The drawing under review shows one solid part. Ordinate dimensions are in mm from its lowest x, y, z. Round coordinates to 2 decimals unless told otherwise and drop trailing zeros. Write each loop counter-clockwise with the first axis right and the second up, starting at its lowest first coordinate (ties: lowest second). Pieces come first, ordered by that corner, then holes. Notation, with made-up numbers: (-5, 62.5) -> (11, 62.5) arc R24 cw to (11, 92.5) -> close; hole circle Ø10 at (54.5, -3). An arc over 180 degrees is marked (long way). Answer in a Markdown table with one row per item.
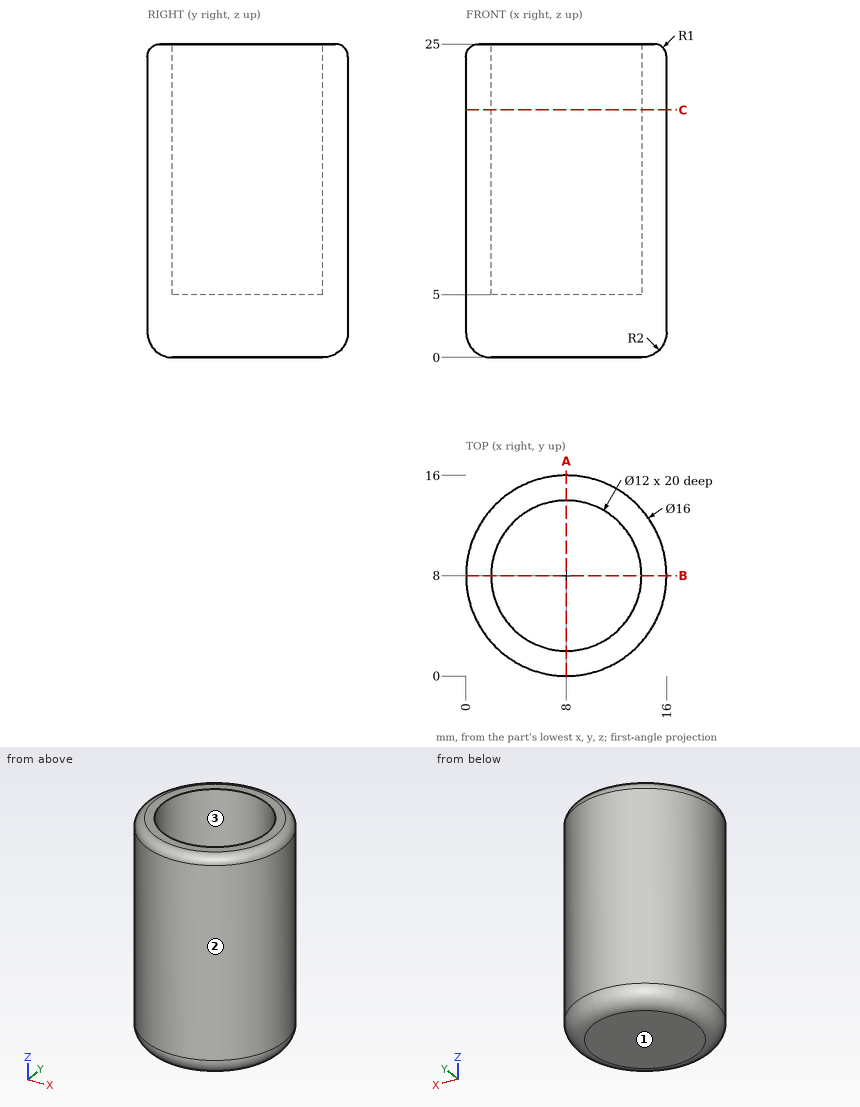
1) Mouldability with a two-part tool opening along Y and no side actions: class the marked faces 1, 2 and 3 as pulls with the +Y half, pulls with the -Y half, needs draft (parallel to the pull), parting line crosses it, or undercut.
Solved:
| item | result |
|---|---|
| face 1 | needs draft |
| face 2 | parting line crosses it |
| face 3 | undercut |
2) Clearance check with flat-ended pins moving along their axes: pin 1 Ø1.5 at (y, z) = (10.5, 10.5) entering from -X; pin 2 Ø5 at (x, y) = (2, 12) entering from -Z; pin 3 Ø6 at (x, z) = (13.5, 6) entering from +Y; pin 4 Ø2 at (x, z) = (14.5, 16.5) entering from +Y. State where each tip first meets the part, or that it passes through.
Solved:
| item | result |
|---|---|
| pin 1 | x = 0.19 |
| pin 2 | z = 0 |
| pin 3 | y = 15.6 |
| pin 4 | y = 13.81 |
3) Consider section A-A on x = 8. State the section outline as (y, z) points, then the cut area to 3 significant figures.
Solved:
| item | result |
|---|---|
| outline | (0, 2) arc R2 ccw to (2, 0) -> (14, 0) arc R2 ccw to (16, 2) -> (16, 24) arc R1 ccw to (15, 25) -> (14, 25) -> (14, 5) -> (2, 5) -> (2, 25) -> (1, 25) arc R1 ccw to (0, 24) -> close |
| area | 158 mm² |
4) For line 1 (Y direction, x = 8, z = 20.75); line 2 (Z direction, x = 4.5, y = 10); line 3 (Y direction, x = 13, z = 13.25) (3 decimals), list the stretches that pass through material, from the lowest coordinate up. Write a range as [from, to].
Solved:
| item | result |
|---|---|
| line 1 | [0, 2], [14, 16] |
| line 2 | [0, 5] |
| line 3 | [1.755, 4.683], [11.317, 14.245] |
5) Consider section C-C on z = 19.75. State the section outline as (x, y) points, then the cut area to 3 significant figures.
Solved:
| item | result |
|---|---|
| outline | circle Ø16 at (8, 8); hole circle Ø12 at (8, 8) |
| area | 88.0 mm² |
